```python
from build123d import *

# Parameters (mm, degrees)
BOSS_EXTRU_1_DEPTH = 30


with BuildPart() as part:
    # Esquisse1 → Boss.-Extru.1 (new body)
    with BuildSketch(Plane.XY):
        with BuildLine():
            Line((46.368433326, 259.570837519), (46.368433326, 263.007656324))
            Line((46.368433326, 263.007656324), (50, 263.007656324))
            ThreePointArc((50, 263.007656324), (159.652687148, 23.346633699), (99.977310085, -233.363254962))
            ThreePointArc((99.977310085, -233.363254962), (-1.517561323, -281.361033685), (-104.221114809, -236.007138747))
            ThreePointArc((-104.221114809, -236.007138747), (-164.627534347, 23.847528243), (-53.631566674, 266.444475128))
            Line((-53.631566674, 266.444475128), (-50, 266.444475128))
            Line((-50, 266.444475128), (-50, 263.007656324))
            ThreePointArc((-50, 263.007656324), (-159.652687148, 23.346633699), (-99.977310085, -233.363254962))
            ThreePointArc((-99.977310085, -233.363254962), (-1.526330683, -276.127902533), (95.733505362, -230.719371177))
            ThreePointArc((95.733505362, -230.719371177), (154.677839949, 22.845739156), (46.368433326, 259.570837519))
        make_face()
    extrude(amount=BOSS_EXTRU_1_DEPTH)


solid = part.part
```
Model file for the job. Use its own axes, mm. A direction names the side the tool comes from. Coordinates: 2 decimals unless noted, no trailing zeros. Loops run counter-clockwise (first coordinate to the right, second up) from the corner with the lowest first, then second, coordinate; pieces in that order, holes last. Notation, with made-up numbers: (-5.5, 61) - (39.5, 61) arc R15 ccw to (39.5, 70) - close; hole circle Ø11 at (44, 47.5). An arc over 180 degrees is marked (long way). Write item = value, one per line. Start each with the question number.
Item 1: Pull direction X, two halves, no side cores. Call faces 1 (the face through (-159.26, 27.08, 14.79)), 2 (the face through (-164.99, 20.06, 14.79)), 3 (the face through (0.1, -281.33, 14.79)), 4 (the face through (-3.07, -276.14, 14.79)): +X half, -X half, draft (parallel to the pull), parting line (faces both ways), or undercut.
Item 2: Drop flat-ended pins along their axis: pin 1 Ø5 at (x, z) = (-59, 5) entering from +Y; pin 2 Ø1.8 at (x, z) = (49, 21.5) entering from +Y; pin 3 Ø3 at (x, z) = (102, 3.5) entering from +Y. Give the stop position or say it passes through.
Item 3: Wall check: probe 1 along X at (y, z) = (-22.5, 19); probe 2 along Y at (x, z) = (1.5, 22.5); probe 3 along X at (y, z) = (-152, 20.25). Give the ranges that are in metal, low to high. Write a range as [from, to].
Item 4: Saw through at C-C, the plane z = 12. List the corners of the cut face in (x, y), then the cut area to 3 significant figures.
Item 5: Saw through at D-D, the plane x = -4.5. List the corners of the cut face in (y, z), then the cut area to 3 significant figures.
Item 6: 3-axis set-ups, long thin cutter, end or side, ignore diameter. For faces 5 (the face through (159.26, 27.08, 14.79)), 6 (the face through (155.033, 19.152, 14.79)): which of +Z, -Z, +X, -X, +Y, -Y reach the whole face in a straight line?
Item 7: Saw through at B-B, the plane y = -93.5. List the corners of the cut face in (x, z).
Item 8: Saw through at A-A, the plane x = 70.5. List the corners of the cut face in (y, z), then the cut area to 3 significant figures.
Answers:
q1.face_1 = undercut
q1.face_2 = -X half
q1.face_3 = parting line
q1.face_4 = undercut
q2.pin_1 = 263.38
q2.pin_2 = 263.01
q2.pin_3 = 197.44
q3.probe_1 = [-166.68, -161.68], [156.68, 161.68]
q3.probe_2 = [-281.29, -276.05]
q3.probe_3 = [-144.21, -138.92], [133.62, 138.92]
q4.outline = (-104.22, -236.01) arc R135.02 ccw to (99.98, -233.36) arc R408.15 ccw to (50, 263.01) - (46.37, 263.01) - (46.37, 259.57) arc R403.15 cw to (95.73, -230.72) arc R130.66 cw to (-99.98, -233.36) arc R408.15 cw to (-50, 263.01) - (-50, 266.44) - (-53.63, 266.44) arc R413.15 ccw to start
q4.area = 6,540 mm2
q5.outline = (-281.37, 0) - (-276.13, 0) - (-276.13, 30) - (-281.37, 30) - close
q5.area = 157 mm2
q6.face_5 = +Z, -Z, +X
q6.face_6 = +Z, -Z
q7.outline = (-159.66, 0) - (-154.58, 0) - (-154.58, 30) - (-159.66, 30) - close; (149.49, 0) - (154.58, 0) - (154.58, 30) - (149.49, 30) - close
q8.outline = (-259.44, 0) - (-253.31, 0) - (-253.31, 30) - (-259.44, 30) - close; (231.61, 0) - (239.62, 0) - (239.62, 30) - (231.61, 30) - close
q8.area = 424 mm2
